Model file for the job. Use its own axes, mm. A direction names the side the tool comes from. Give positions to 0.01 mm unless a question says otherwise; leave off trailing zeros. Write each loop counter-clockwise with the first axis right and the second up, starting at its lowest first coordinate (ties: lowest second). Pieces come first, ordered by that corner, then holes. Notation, with made-up numbers: (44.5, 15.25) - (88.5, 15.25) arc R9 ccw to (88.5, 30.25) - close; hole circle Ø4 at (53, 24.5). An arc over 180 degrees is marked (long way). One line per item, written item: value. Start each with the question number.
(1) Probe L1, parallel to Y at x = 3.75, z = 0; L2, parallel to Y at x = -7, z = -1.25; L3, parallel to X at y = 7, z = 3. List the from-to ranges inside material, lowest first.
(2) Cut at C-C, the plane z = 5.25. List the corners of the cut face in (x, y), and give its area (4 significant figures).
(3) Cut at D-D, the plane x = -6.5. List the corners of the cut face in (y, z).
(4) Cut at A-A, the plane z = 0. List the corners of the cut face in (x, y).
(5) Cut at B-B, the plane x = 0. List the corners of the cut face in (y, z), and give its area (3 significant figures).
(6) 3-axis set-ups, long thin cutter, end or side, ignore diameter. For faces 4 (the face through (-2, 0, -3)), 5 (the face through (0, 50, 0)), 6 (the face through (-0.867, -2.465, -3.905)): which of +Z, -Z, +X, -X, +Y, -Y reach the whole face in a straight line?
(7) Drop flat-ended pins along their axis: P1, Ø10, axis at y = 2, z = -0.5, coming from the -X side; P2, Ø5, axis at y = 5.5, z = 6, coming from the +X side; P3, Ø6, axis at x = -5.5, z = 4.5, coming from the -Y side; P4, Ø8, axis at y = 2, z = -3, coming from the +X side. Give the stop position or say it passes through.
(8) Mould opens along Y. For faces 1 (the face through (-0.73, 12.32, -3.29)), 2 (the face through (0, 37, -9.3)), 3 (the face through (0, -5, 0)) say: pulls with the +Y half, pulls with the -Y half, needs draft (parallel to the pull), parting line crosses it, or undercut.
from build123d import *

# Parameters (mm, degrees)
F0_R     = 4
F1_DEPTH = 5
F2_R     = 3.370831
F3_DEPTH = 25
F4_W     = 18.300004
F4_H     = 18.600002
F5_DEPTH = 25


with BuildPart() as f1:
    # F0 (on Front) → F1 (new body)
    with BuildSketch(Plane.XZ):
        Circle(F0_R)
    extrude(amount=F1_DEPTH)

    # F2 (on Front) → F3 (join)
    with BuildSketch(Plane.XZ):
        Circle(F2_R)
    extrude(amount=-F3_DEPTH)

    # F4 (on face) → F5 (join)
    with BuildSketch(Plane(origin=(0, 25, 0), x_dir=(-1, 0, 0), z_dir=(0, 1, 0))):
        Rectangle(F4_W, F4_H)
    extrude(amount=F5_DEPTH)


solid = f1.part
Answers follow:
1. L1: y = -5 to 0, 25 to 50
1. L2: y = 25 to 50
1. L3: x = -1.54 to 1.54
2. outline: (-9.15, 25) - (9.15, 25) - (9.15, 50) - (-9.15, 50) - close
2. area: 457.5 mm²
3. outline: (25, -9.3) - (50, -9.3) - (50, 9.3) - (25, 9.3) - close
4. outline: (-9.15, 25) - (-3.37, 25) - (-3.37, 0) - (-4, 0) - (-4, -5) - (4, -5) - (4, 0) - (3.37, 0) - (3.37, 25) - (9.15, 25) - (9.15, 50) - (-9.15, 50) - close
5. outline: (-5, -4) - (0, -4) - (0, -3.37) - (25, -3.37) - (25, -9.3) - (50, -9.3) - (50, 9.3) - (25, 9.3) - (25, 3.37) - (0, 3.37) - (0, 4) - (-5, 4) - close
5. area: 674 mm²
6. face 4: none
6. face 5: +Z, -Z, +X, -X, +Y
6. face 6: -Y
7. P1: stops at x = -4
7. P2: passes through
7. P3: stops at y = 25
7. P4: stops at x = 4
8. face 1: undercut
8. face 2: needs draft
8. face 3: pulls with the -Y half
